Autodesk Inventor part; units mm, degrees
ref_plane "Start plane" through (0, 0, 50) normal (0, 0, 1) x (1, 0, 0)
ref_plane "End plane" through (0, 0, 1632) normal (0, 0, 1) x (1, 0, 0)
ref_plane "Work Plane4" through (9.2, 45, 1632) normal (0, 0, 1) x (1, 0, 0)
ref_plane "Start plane" through (0, 0, 50) normal (0, 0, 1) x (1, 0, 0)
ref_plane "End plane" through (0, 0, 1632) normal (0, 0, 1) x (1, 0, 0)
sketch "Sketch" plane through (0, 0, 0) normal (0, 0, 1) x (1, 0, 0)
  line L0 (-15, -11.25) -> (-15, 11.25)
  line L1 (-11.25, 15) -> (11.25, 15)
  line L2 (15, 11.25) -> (15, -11.25)
  line L3 (11.25, -15) -> (-11.25, -15)
  arc A0 (-15, -11.25) -> (-11.25, -15) centre (-11.25, -11.25) ccw
  arc A1 (-11.25, 15) -> (-15, 11.25) centre (-11.25, 11.25) ccw
  arc A2 (15, 11.25) -> (11.25, 15) centre (11.25, 11.25) ccw
  arc A3 (11.25, -15) -> (15, -11.25) centre (11.25, -11.25) ccw
  arc A4 (-11.25, 12.5) -> (-12.5, 11.25) centre (-11.25, 11.25) ccw
  line L4 (-11.25, 12.5) -> (11.25, 12.5)
  arc A5 (12.5, 11.25) -> (11.25, 12.5) centre (11.25, 11.25) ccw
  line L5 (12.5, 11.25) -> (12.5, -11.25)
  arc A6 (11.25, -12.5) -> (12.5, -11.25) centre (11.25, -11.25) ccw
  line L6 (11.25, -12.5) -> (-11.25, -12.5)
  arc A7 (-12.5, -11.25) -> (-11.25, -12.5) centre (-11.25, -11.25) ccw
  line L7 (-12.5, -11.25) -> (-12.5, 11.25)
  line L8 (0, 22.0873) -> (0, -22.0873) construction
  line L9 (-22.0873, 0) -> (22.0873, 0) construction
  dimension "d7" = 3.75
  dimension "d10" = 30
  dimension "d11" = 30
  dimension "d12" = 2.5
  dimension "d15" = 15
  dimension "d16" = 15
extrude "Body" add sketch "Sketch" along normal up to surface (1582 mm away) from surface at 50
sketch "Sketch3" plane through (0, 0, 0) normal (0, 0, 1) x (1, 0, 0)
  line L0 (0, 0) -> (10, 0)
ref_plane "Work Plane3" through (0, 0, 0) normal (0, -1, 0) x (1, 0, 0)
sketch "Sketch4" plane through (0, 0, 0) normal (0, -1, 0) x (1, 0, 0)
  line L0 (-2, 50) -> (12, 50)
  line L1 (-2, 1632) -> (12, 1632)
  dimension "d18" = 1582
ref_plane "Work Plane4" through (9.2, 45, 1632) normal (0, 0, 1) x (1, 0, 0)
split "Split1" plane through (9.2, 45, 1632) removes the side toward (0, 0, 1)
ref_plane "Work Plane5" through (-629.2, 45, 50) normal (0, 0, -1) x (-1, 0, 0)
split "Split2" plane through (-629.2, 45, 50) removes the side toward (0, 0, -1)
ref_plane "Work Plane6" through (-630.2, -705, 1632) normal (0, 0, 1) x (1, 0, 0)
split "Split3" plane through (-630.2, -705, 1632) removes the side toward (0, 0, 1)
equation "\"d7\" = G_IR"
equation "\"d10\" = G_H"
equation "\"d11\" = G_W"
equation "\"d12\" = G_T"
equation "\"d15\" = 0.5 * d10"
equation "\"d16\" = 0.5 * d11"
equation "\"d3\" = G_L"
equation "\"G_W\" = 30"
equation "\"G_H\" = 30"
equation "\"G_T\" = 2.5"
equation "\"G_IR\" = 3.75"
equation "\"G_L\" = d18"
equation "\"d14\" = G_OFFSET_END + B_L"
equation "\"B_L\" = 1682"
properties part number "DIN EN 10305-5 - 30 x 30 x 2,5  - 1582" material "Steel, Mild"
CAD build for the part. Positions are in the model's coordinates, mm. Round coordinates to 2 decimals unless told otherwise and drop trailing zeros. Order: outer loops, then holes, each group sorted by start corner. A loop starts at its lowest first (then second) coordinate and runs counter-clockwise, first axis right, second up.
Q1. Wall check: L1, parallel to Y at x = 12, z = 1195.5; L2, parallel to X at y = 1, z = 1409.5. Give the ranges that are in metal, low to high.
Q2. Slice it at B-B (z = 567). Write the cut outline in (x, y), and give its area (3 significant figures).
Q3. Slice it at A-A (x = 6). Write the cut outline in (y, z).
Q4. Drop flat-ended pins along their axis: pin 1 (5 mm diameter, centred on x = 8.5, y = -5.5, fed in from +Z); pin 2 (4 mm diameter, centred on x = 6.5, y = -12, fed in from +Z). Give the stop position or say it passes through.
Results below:
1. L1: y = -14.92 to -12.25, 12.25 to 14.92
1. L2: x = -15 to -12.5, 12.5 to 15
2. outline: (-15, -11.25) arc R3.75 ccw to (-11.25, -15) - (11.25, -15) arc R3.75 ccw to (15, -11.25) - (15, 11.25) arc R3.75 ccw to (11.25, 15) - (-11.25, 15) arc R3.75 ccw to (-15, 11.25) - close; hole (-12.5, -11.25) arc R1.25 ccw to (-11.25, -12.5) - (11.25, -12.5) arc R1.25 ccw to (12.5, -11.25) - (12.5, 11.25) arc R1.25 ccw to (11.25, 12.5) - (-11.25, 12.5) arc R1.25 ccw to (-12.5, 11.25) - close
2. area: 264 mm2
3. outline: (-15, 50) - (-12.5, 50) - (-12.5, 1632) - (-15, 1632) - close; (12.5, 50) - (15, 50) - (15, 1632) - (12.5, 1632) - close
4. pin 1: passes through
4. pin 2: stops at z = 1632
